from build123d import *

# Parameters (mm, degrees)
BOX002002_W     = 22
BOX002002_H     = 24
BOX002002_DEPTH = 13
BOX002_W        = 19
BOX002_H        = 34
BOX002_DEPTH    = 28
BOX002001_W     = 21
BOX002001_H     = 38
BOX002001_DEPTH = 32


with BuildPart() as box002002:
    # Box002002 → Box002002 (new body)
    with BuildSketch(Plane.XY.offset(2)):
        with Locations((11, 12)):
            Rectangle(BOX002002_W, BOX002002_H)
    extrude(amount=BOX002002_DEPTH)


with BuildPart() as fusion007:
    # Box002 → Box002 (new body)
    with BuildSketch(Plane(origin=(0, -5, 2), x_dir=(1, 0, 0), z_dir=(0, 0, 1))):
        with Locations((9.5, 17)):
            Rectangle(BOX002_W, BOX002_H)
    extrude(amount=BOX002_DEPTH)

    # Fusion007: union Box002002
    add(box002002.part)


with BuildPart() as cut:
    # Box002001 → Box002001 (new body)
    with BuildSketch(Plane(origin=(0, -7, 0), x_dir=(1, 0, 0), z_dir=(0, 0, 1))):
        with Locations((10.5, 19)):
            Rectangle(BOX002001_W, BOX002001_H)
    extrude(amount=BOX002001_DEPTH)

    # Cut: cut Fusion007
    add(fusion007.part, mode=Mode.SUBTRACT)


solid = cut.part
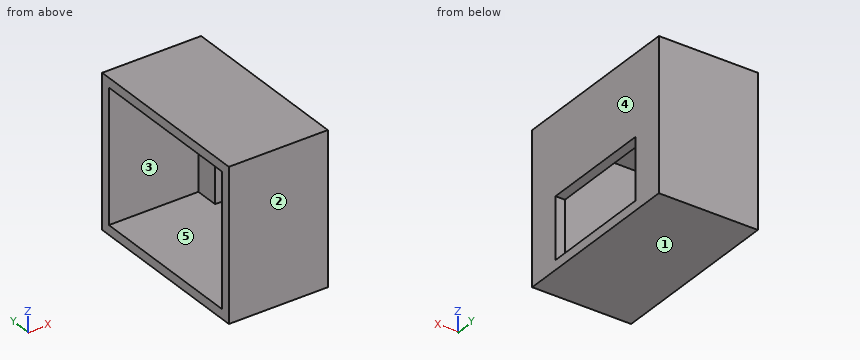
For this review, take the finished solid that the model builds, in its own axes (mm). Face numbers are marked on the shaded views. A direction names the side the tool comes from. Coordinates: 2 decimals unless noted, no trailing zeros. Write each loop counter-clockwise with the first axis right and the second up, starting at its lowest first coordinate (ties: lowest second). Pieces come first, ordered by that corner, then holes. Notation, with made-up numbers: (41.25, 41.25) -> (51.25, 41.25) arc R22 ccw to (51.25, 67.25) -> close; hole circle Ø8 at (-15.75, 62.25). An arc over 180 degrees is marked (long way). Write each question's results on one line, items separated by ' | '. Start each with the question number.
1) Consider section D-D (y = 28). Write out the cut boundary in (x, z), plus the area to 3 significant figures.
2) For the marked faces 4 and 5, list the 3-axis set-ups (+Z, -Z, +X, -X, +Y, -Y) from which the entire face can be reached by the end or side of a thin tool; tool diameter is ignored.
3) Wall thickness on L1, parallel to Y at x = 12.5, z = 12; L2, parallel to Z at x = 8.5, y = 12; L3, parallel to X at y = 11, z = 23: over which ranges is each line inside the solid? List them lowest first. Write a range as [from, to].
4) Consider section C-C (y = 17.5). Write out the cut boundary in (x, z).
5) The part is to be moulded in two halves that separate along Y. For the marked faces 1, 2 and 3, say which applies: +Y half, -Y half, draft (parallel to the pull), parting line (faces both ways), or undercut.
6) Consider section A-A (z = 10). Write out the cut boundary in (x, y), plus the area to 3 significant figures.
7) Insertion check: pin 1 (14 mm diameter, centred on y = 19, z = 18, fed in from -X). The pin has a flat end and moves straight along its axis. Give the tip position at first contact, or say it passes through.
8) Consider section B-B (x = 17). Write out the cut boundary in (y, z).
Geometry says:
1) outline: (0, 0) -> (21, 0) -> (21, 32) -> (0, 32) -> (0, 30) -> (19, 30) -> (19, 2) -> (0, 2) -> close | area: 140 mm^2
2) face 4: +Z, -Z, +X, +Y, -Y | face 5: -X
3) L1: [-7, -5], [29, 31] | L2: [0, 2], [30, 32] | L3: [19, 21]
4) outline: (0, 0) -> (21, 0) -> (21, 2) -> (0, 2) -> close; (0, 30) -> (19, 30) -> (19, 15) -> (21, 15) -> (21, 32) -> (0, 32) -> close
5) face 1: draft | face 2: -Y half | face 3: undercut
6) outline: (0, -7) -> (21, -7) -> (21, 0) -> (19, 0) -> (19, -5) -> (0, -5) -> close; (0, 29) -> (19, 29) -> (19, 24) -> (21, 24) -> (21, 31) -> (0, 31) -> close | area: 104 mm^2
7) pin 1: x = 19
8) outline: (-7, 0) -> (31, 0) -> (31, 32) -> (-7, 32) -> close; hole (-5, 2) -> (29, 2) -> (29, 30) -> (-5, 30) -> close
